Can you work these out from the model? Positions are in its coordinate system, mm. Face numbers are marked on the shaded views. Give positions to 0.01 mm unless a question says otherwise; leave off trailing zeros. Loops run counter-clockwise (first coordinate to the right, second up) from the corner with the lowest first, then second, coordinate; pieces in that order, holes last. Notation, with made-up numbers: (-29, 40) - (6, 40) arc R31 ccw to (6, 78) - close; hole circle Ø10 at (80, -29). An arc over 180 degrees is marked (long way). Answer as a JSON object with one key per item and string values. Group by question number.
Item 1: Suppose I cut it at B-B on x = -4.5. Count the separate pieces of the cut face and the enclosed holes in it, and give its area (3 significant figures).
Item 2: Suppose I cut it at C-C on y = -2.5. Write out the boundary of the cut face in (x, z), and give its area (3 significant figures).
Item 3: Please list where these lines run through material, in increasing order: L1, parallel to Z at x = -24, y = -7; L2, parallel to Y at x = -24.5, z = 7; L3, parallel to X at y = -7.75, z = -11.5.
Item 4: Suppose I cut it at A-A on x = 8. Write out the boundary of the cut face in (y, z).
Item 5: Thinking about a two-plate mould opening in Y: for the marked faces 1, 2, 3 and 4, which applies, pulls with the +Y half, pulls with the -Y half, needs draft (parallel to the pull), parting line crosses it, or undercut?
Item 6: Suppose I cut it at D-D on z = -10.5. Write out the boundary of the cut face in (x, y), and give its area (3 significant figures).
Item 7: Will this pin go through, and if not, where does the flat tip stop? pin 1 (3 mm diameter, centred on y = -6, z = 10.5, fed in from +X).
from build123d import *

# Parameters (mm, degrees)
F0_R     = 2.54
F0_W     = 25.4
F0_H     = 25.4
F1_DEPTH = 12.7
F2_W     = 9.547732
F2_H     = 73.135637
F3_DEPTH = 71.12


with BuildPart() as f1:
    # F0 (on Front) → F1 (new body)
    with BuildSketch(Plane.XZ):
        Polygon((-18.806005, 40.205049), (-44.206005, 40.205049), (-44.206005, 14.805049), (-40.768821, 14.805049), (-18.806005, 14.805049), align=None)
        with Locations((-31.506005, 27.505049)):
            Circle(F0_R, mode=Mode.SUBTRACT)
        Polygon((-40.768821, 14.805049), (-44.206005, 14.805049), (-44.206005, -10.594951), (-18.806005, -10.594951), (-18.806005, 14.805049), align=None)
        with Locations((-31.506005, 2.105049)):
            Circle(F0_R, mode=Mode.SUBTRACT)
        with Locations((-6.106005, 27.505049)):
            Rectangle(F0_W, F0_H)
        with Locations((-6.106005, 27.505049)):
            Circle(F0_R, mode=Mode.SUBTRACT)
        with Locations((-31.506005, -23.294951)):
            Rectangle(F0_W, F0_H)
        with Locations((-31.506005, -23.294951)):
            Circle(F0_R, mode=Mode.SUBTRACT)
        with Locations((19.293995, 27.505049)):
            Rectangle(F0_W, F0_H)
        with Locations((19.293995, 27.505049)):
            Circle(F0_R, mode=Mode.SUBTRACT)
        with Locations((-6.106005, -23.294951)):
            Rectangle(F0_W, F0_H)
        with Locations((-6.106005, -23.294951)):
            Circle(F0_R, mode=Mode.SUBTRACT)
        with Locations((19.293995, 2.105049)):
            Rectangle(F0_W, F0_H)
        with Locations((19.293995, 2.105049)):
            Circle(F0_R, mode=Mode.SUBTRACT)
        with Locations((19.293995, -23.294951)):
            Rectangle(F0_W, F0_H)
        with Locations((19.293995, -23.294951)):
            Circle(F0_R, mode=Mode.SUBTRACT)
        with Locations((-6.106005, 2.105049)):
            Rectangle(F0_W, F0_H)
        with Locations((-6.106005, 2.105049)):
            Circle(F0_R, mode=Mode.SUBTRACT)
    extrude(amount=F1_DEPTH)

    # F2 (on face) → F3 (cut)
    with BuildSketch(Plane.YZ.offset(31.993995)):
        with Locations((-6.396981, 2.100502)):
            Rectangle(F2_W, F2_H)
    extrude(amount=-F3_DEPTH, mode=Mode.SUBTRACT)


solid = f1.part
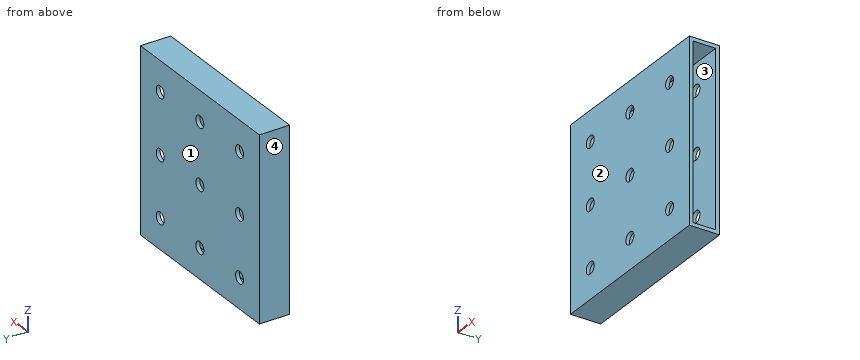
Worked out:
{
 "1": {"separate pieces": "6", "enclosed holes": "0", "area": "232 mm2"},
 "2": {"outline": "(-44.21, -35.99) - (31.99, -35.99) - (31.99, -34.47) - (-39.13, -34.47) - (-39.13, 38.67) - (31.99, 38.67) - (31.99, 40.21) - (-44.21, 40.21) - close", "area": "605 mm2"},
 "3": {"L1": "z = -35.99 to -34.47, 38.67 to 40.21", "L2": "y = -12.7 to -11.17, -1.62 to 0", "L3": "x = -44.21 to -39.13"},
 "4": {"outline": "(-12.7, -35.99) - (0, -35.99) - (0, 40.21) - (-12.7, 40.21) - close; hole (-11.17, -34.47) - (-1.62, -34.47) - (-1.62, 38.67) - (-11.17, 38.67) - close"},
 "5": {"face 1": "pulls with the +Y half", "face 2": "pulls with the -Y half", "face 3": "undercut", "face 4": "needs draft"},
 "6": {"outline": "(-44.21, -12.7) - (31.99, -12.7) - (31.99, -11.17) - (-39.13, -11.17) - (-39.13, -1.62) - (31.99, -1.62) - (31.99, 0) - (-44.21, 0) - close", "area": "289 mm2"},
 "7": {"pin 1": "stops at x = -39.13"}
}
